```python
from build123d import *

# Parameters (mm, degrees)
F0_R     = 57.0036586855
F0_R_2   = 10.16
F1_DEPTH = 3.175
F2_SIZE  = 3.175
F3_SIZE  = 3.17499


# Not quite as in the source:
# - a fillet or chamfer is up to 0.001 mm smaller than in the source, because OpenCascade refuses the exact size


with BuildPart() as f1:
    # F0 (on Front) → F1 (new body, symmetric)
    with BuildSketch(Plane.XZ):
        Circle(F0_R)
        Circle(F0_R_2, mode=Mode.SUBTRACT)
    extrude(amount=F1_DEPTH, both=True)

    # F2
    f2_edges = [f1.edges().sort_by_distance(p)[0] for p in [
        (-57.003659, 3.175, 0),
    ]]
    chamfer(f2_edges, length=F2_SIZE)

    # F3 (size 3.175 in the source; OpenCascade refuses exactly that, so slightly less here)
    f3_edges = [f1.edges().sort_by_distance(p)[0] for p in [
        (-57.003659, -3.175, 0),
    ]]
    chamfer(f3_edges, length=F3_SIZE)


solid = f1.part
```
Here's how the part is built. I have some questions about the finished solid (model axes, mm). Give positions to 0.01 mm unless a question says otherwise; leave off trailing zeros. Loops run counter-clockwise (first coordinate to the right, second up) from the corner with the lowest first, then second, coordinate; pieces in that order, holes last. Notation, with made-up numbers: M 28,41 L 87,41 A28 ccw 87,77 Z; hole C -8.5,39 d8. An arc over 180 degrees is marked long. Put each result on its own line as item: value. Start each with the question number.
(1) I need wall thicknesses on line 1 along Z through (x, y) = (5, 2); line 2 along Z through (x, y) = (0, -1.25); line 3 along Z through (x, y) = (-34, 0.25). Which ranges of each line are inside material? Lowest first, please. Write a range as [from, to].
(2) I want a section at C-C on y = -1.75. Please give me the cut outline in (x, z), then the cut area to 3 significant figures.
(3) Will these pins go through, and if not, where does the flat tip stop? pin 1 Ø1.5 at (y, z) = (2.5, -35) entering from -X; pin 2 Ø12 at (x, z) = (0, 0) entering from -Y; pin 3 Ø2 at (y, z) = (1.5, -25.5) entering from -X.
Answer block:
1. line 1: [-54.78, -8.84], [8.84, 54.78]
1. line 2: [-55.75, -10.16], [10.16, 55.75]
1. line 3: [-45.44, 45.44]
2. outline: C 0,0 d110.51; hole C 0,0 d20.32
2. area: 9,270 mm^2
3. pin 1: x = -42.93
3. pin 2: through
3. pin 3: x = -50.53
